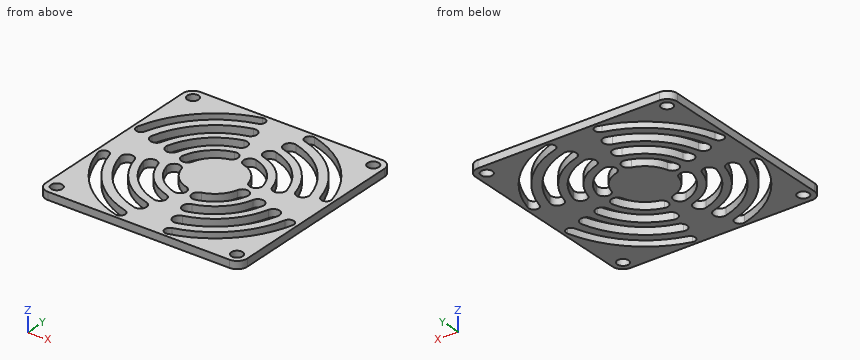
Autodesk Inventor part; units mm, degrees
ref_plane "YZ Plane" through (0, 0, 0) normal (1, 0, 0) x (0, 1, 0)
ref_plane "XZ Plane" through (0, 0, 0) normal (0, 1, 0) x (-1, 0, 0)
ref_plane "XY Plane" through (0, 0, 0) normal (0, 0, 1) x (1, 0, 0)
sketch "Sketch1" plane through (0, 0, 0) normal (0, 0, 1) x (1, 0, 0)
  line L0 (-40, -40) -> (40, -40)
  line L1 (40, -40) -> (40, 40)
  line L2 (40, 40) -> (-40, 40)
  line L3 (-40, 40) -> (-40, -40)
  line L4 (-40, -40) -> (40, 40) construction
  line L5 (40, -40) -> (-40, 40) construction
  point P0 (0, 0)
  dimension "d0" = 80
  dimension "d1" = 80
extrude "Extrusion1" add sketch "Sketch1" along normal blind 3
sketch "Sketch2" plane through (0, 0, 3) normal (0, 0, 1) x (1, 0, 0)
  arc A0 (-9.8351, 36.7052) -> (-36.7052, 9.8351) centre (0, 0) ccw construction
  arc A1 (-10.3528, 38.637) -> (-38.637, 10.3528) centre (0, 0) ccw
  arc A2 (-9.3175, 34.7733) -> (-34.7733, 9.3175) centre (0, 0) ccw
  arc A3 (-9.3175, 34.7733) -> (-10.3528, 38.637) centre (-9.8351, 36.7052) ccw
  arc A4 (-38.637, 10.3528) -> (-34.7733, 9.3175) centre (-36.7052, 9.8351) ccw
  arc A5 (-7.7646, 28.9778) -> (-28.9778, 7.7646) centre (0, 0) ccw construction
  arc A6 (-8.4116, 31.3926) -> (-31.3926, 8.4116) centre (0, 0) ccw
  arc A7 (-7.1175, 26.563) -> (-26.563, 7.1175) centre (0, 0) ccw
  arc A8 (-7.1175, 26.563) -> (-8.4116, 31.3926) centre (-7.7646, 28.9778) ccw
  arc A9 (-31.3926, 8.4116) -> (-26.563, 7.1175) centre (-28.9778, 7.7646) ccw
  arc A10 (-5.694, 21.2504) -> (-21.2504, 5.694) centre (0, 0) ccw construction
  arc A11 (-6.3411, 23.6652) -> (-23.6652, 6.3411) centre (0, 0) ccw
  arc A12 (-5.047, 18.8356) -> (-18.8356, 5.047) centre (0, 0) ccw
  arc A13 (-5.047, 18.8356) -> (-6.3411, 23.6652) centre (-5.694, 21.2504) ccw
  arc A14 (-23.6652, 6.3411) -> (-18.8356, 5.047) centre (-21.2504, 5.694) ccw
  line L0 (0, 0) -> (-62.4866, 0) construction
  line L1 (0, 0) -> (-61.1079, 16.3738) construction
  line L2 (0, 0) -> (0, 46.5462) construction
  line L3 (0, 0) -> (-12.1401, 45.3074) construction
  arc A15 (-3.6235, 13.523) -> (-13.523, 3.6235) centre (0, 0) ccw construction
  arc A16 (-4.2705, 15.9378) -> (-15.9378, 4.2705) centre (0, 0) ccw
  arc A17 (-2.9764, 11.1081) -> (-11.1081, 2.9764) centre (0, 0) ccw
  arc A18 (-2.9764, 11.1081) -> (-4.2705, 15.9378) centre (-3.6235, 13.523) ccw
  arc A19 (-15.9378, 4.2705) -> (-11.1081, 2.9764) centre (-13.523, 3.6235) ccw
  dimension "d4" = 38
  dimension "d5" = 15
  dimension "d6" = 15
  dimension "d7" = 30
  dimension "d8" = 22
  dimension "d9" = 4
  dimension "d10" = 5
  dimension "d11" = 5
  dimension "d12" = 14
  dimension "d13" = 5
extrude "Extrusion2" cut sketch "Sketch2" against normal blind 3
pattern_circular "Circular Pattern1" count 4 over 360 about axis through (0, 0, -10) along (0, 0, 1) of "Extrusion2"
sketch "Sketch3" plane through (0, 0, 3) normal (0, 0, 1) x (1, 0, 0)
  line L0 (-35.75, -35.75) -> (35.75, -35.75) construction
  line L1 (35.75, -35.75) -> (35.75, 35.75) construction
  line L2 (35.75, 35.75) -> (-35.75, 35.75) construction
  line L3 (-35.75, 35.75) -> (-35.75, -35.75) construction
  line L4 (-35.75, -35.75) -> (35.75, 35.75) construction
  line L5 (35.75, -35.75) -> (-35.75, 35.75) construction
  point P0 (0, 0)
  dimension "d19" = 71.5
  dimension "d20" = 71.5
hole "Hole1" at (-35.75, 35.75, 3) at (35.75, 35.75, 3) at (35.75, -35.75, 3) at (-35.75, -35.75, 3) direction (0, 0, -1) diameter 4.5 depth 8 tip angle 118
fillet "Fillet1" radius 4 4 edges at (-40, 40, 1.5) (-40, -40, 1.5) (40, -40, 1.5) (40, 40, 1.5)
properties part number "Lüftergitter" material "Stainless Steel"
Here's how the part is built. I have some questions about the finished solid (model axes, mm). Round coordinates to 2 decimals unless told otherwise and drop trailing zeros. Order: outer loops, then holes, each group sorted by start corner. A loop starts at its lowest first (then second) coordinate and runs counter-clockwise, first axis right, second up. Notation, with made-up numbers: M 48.5,85.5 L 59.5,85.5 A18 ccw 59.5,106.5 Z; hole C 81,43 d3. An arc over 180 degrees is marked long. Return JSON: item names as keys, results as strings. Group by question number.
1. If we section it at B-B on y = -25.5: List the corners of the cut face in (x, z) for me.
2. If we section it at A-A on y = 21: List the corners of the cut face in (x, z) for me, then the cut area to 3 significant figures.
3. If we section it at C-C on z = 0.45: State how many separate pieces and enclosed holes the cut face has, then the cut area to 3 significant figures.
4. Please list where these lines run through material, in increasing order: probe 1 along X at (y, z) = (-35.75, 1.7); probe 2 along X at (y, z) = (-4, 1.9).
Reply:
{
 "1": {"outline": "M -40,0 L -30.82,0 L -30.82,3 L -40,3 Z; M -25.41,0 L -20.15,0 L -20.15,3 L -25.41,3 Z; M -10.3,0 L 10.3,0 L 10.3,3 L -10.3,3 Z; M 20.15,0 L 25.41,0 L 25.41,3 L 20.15,3 Z; M 30.82,0 L 40,0 L 40,3 L 30.82,3 Z"},
 "2": {"outline": "M -40,0 L -34.04,0 L -34.04,3 L -40,3 Z; M -29.24,0 L -24.8,0 L -24.8,3 L -29.24,3 Z; M -17.76,0 L -12.62,0 L -12.62,3 L -17.76,3 Z; M -3.21,0 L 3.21,0 L 3.21,3 L -3.21,3 Z; M 12.62,0 L 17.76,0 L 17.76,3 L 12.62,3 Z; M 24.8,0 L 29.24,0 L 29.24,3 L 24.8,3 Z; M 34.04,0 L 40,0 L 40,3 L 34.04,3 Z", "area": "112 mm^2"},
 "3": {"separate pieces": "1", "enclosed holes": "20", "area": "4,020 mm^2"},
 "4": {"probe 1": "-40 to -38, -33.5 to -17.94, -8.08 to 8.08, 17.94 to 33.5, 38 to 40", "probe 2": "-40 to -23.09, -19.41 to -15.99, -10.78 to 10.78, 15.99 to 19.41, 23.09 to 40"}
}
